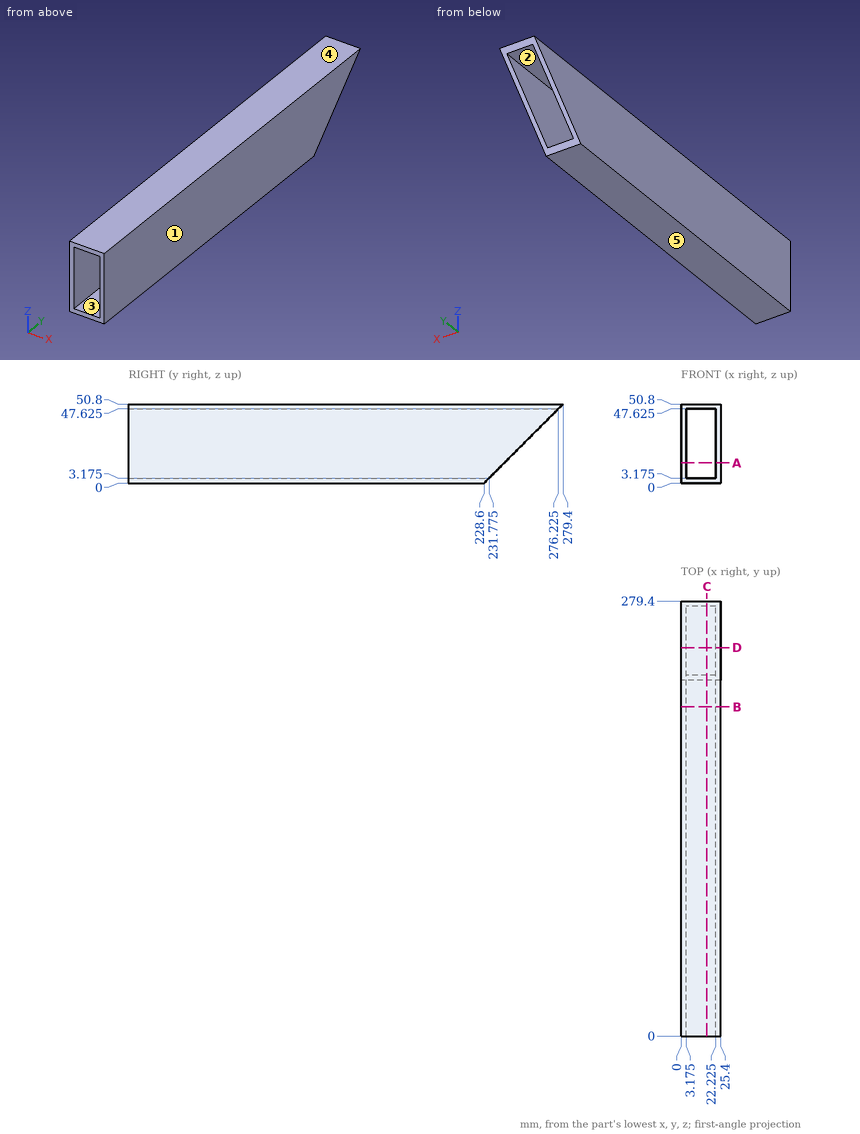
Study the drawing (mm; zero at the part's minimum x, y, z) and answer. A direction names the side the tool comes from. Give positions to 0.01 mm unless a question says otherwise; leave off trailing zeros. Loops run counter-clockwise (first coordinate to the right, second up) from the corner with the lowest first, then second, coordinate; pieces in that order, holes last. Notation, with made-up numbers: (79.25, 88) - (123.25, 88) arc R18 ccw to (123.25, 117) - close; hole circle Ø7 at (34.5, -28). An arc over 180 degrees is marked (long way). Return JSON: item names as keys, results as strings. Group by question number.
1. Find section D-D (y = 249.5). Write down the section's boundary in (x, z) (3 decimals).
2. Find section B-B (y = 211.5). Write down the section's boundary in (x, z) (3 decimals).
3. Find section A-A (z = 13). Write down the section's boundary in (x, y) (3 decimals).
4. Which of the six approach directions +Z, -Z, +X, -X, +Y, -Y give full straight-line access (tool end or side, diameter ignored) to the marked faces 1 and 2?
5. Given pin 1 Ø12 at (x, z) = (12.5, 36) entering from +Y, flat-ended and moving along its own axis, determine where the tip first touches the part or whether it passes through.
6. Determine the mould class of the marked faces 3, 4 and 5 for opening direction Z: pulls with the +Z half, pulls with the -Z half, needs draft (parallel to the pull), parting line crosses it, or undercut.
7. Find section C-C (x = 16.5). Write down the section's boundary in (y, z) (3 decimals), then the cut area to 3 significant figures.
8. Straight lines are drawn through the part: line 1 (X direction, y = 111, z = 10) (3 decimals); line 2 (Z direction, x = 21.75, y = 95.5) (3 decimals); line 3 (Z direction, x = 20.75, y = 244.5) (3 decimals). For each, find the intervals that lie inside material, in ascending order. Write a range as [from, to].
Verdict:
{
 "1": {"outline": "(0, 20.9) - (3.175, 20.9) - (3.175, 47.625) - (22.225, 47.625) - (22.225, 20.9) - (25.4, 20.9) - (25.4, 50.8) - (0, 50.8) - close"},
 "2": {"outline": "(0, 0) - (25.4, 0) - (25.4, 50.8) - (0, 50.8) - close; hole (3.175, 3.175) - (22.225, 3.175) - (22.225, 47.625) - (3.175, 47.625) - close"},
 "3": {"outline": "(0, 0) - (3.175, 0) - (3.175, 241.6) - (0, 241.6) - close; (22.225, 0) - (25.4, 0) - (25.4, 241.6) - (22.225, 241.6) - close"},
 "4": {"face 1": "+Z, -Z, +X, +Y, -Y", "face 2": "+Y, -Y"},
 "5": {"pin 1": "passes through"},
 "6": {"face 3": "undercut", "face 4": "pulls with the +Z half", "face 5": "pulls with the -Z half"},
 "7": {"outline": "(0, 0) - (228.6, 0) - (231.775, 3.175) - (0, 3.175) - close; (0, 47.625) - (276.225, 47.625) - (279.4, 50.8) - (0, 50.8) - close", "area": "1,610 mm^2"},
 "8": {"line 1": "x = [0, 3.175], [22.225, 25.4]", "line 2": "z = [0, 3.175], [47.625, 50.8]", "line 3": "z = [47.625, 50.8]"}
}
